Verification items for the finished model (mm, model axes). Face numbers are marked on the shaded views. Give positions to 0.01 mm unless a question says otherwise; leave off trailing zeros. Order: outer loops, then holes, each group sorted by start corner. A loop starts at its lowest first (then second) coordinate and runs counter-clockwise, first axis right, second up. Notation, with made-up numbers: (-35, -23.75) -> (21, -23.75) arc R17 cw to (21, 6.25) -> close; hole circle Ø10 at (5, 27). An arc over 180 degrees is marked (long way). Write each question's results on one line, items separated by ' | '. Start each with the question number.
1. Cross-section at A-A, the plane y = 32.5. Enter the section's corners in (x, z) (3 decimals), then the cut area to 3 significant figures.
2. Depth check by flat-ended pin: pin 1 Ø1.5 at (y, z) = (56, -0.5) entering from +X; pin 2 Ø4 at (y, z) = (60, 2.5) entering from -X; pin 3 Ø5.5 at (x, z) = (7, -6) entering from -Y. Enter the tip coordinate at first touch or a pass-through.
3. Cross-section at C-C, the plane z = -5. Enter the section's corners in (x, y).
4. Cross-section at B-B, the plane x = 2. Enter the section's corners in (y, z).
5. Cross-section at D-D, the plane y = 46. Enter the section's corners in (x, z) (3 decimals), then the cut area to 3 significant figures.
6. Material ranges on L1, parallel to Z at x = 2, y = 43; L2, parallel to Z at x = 46.5, y = 44; L3, parallel to X at y = 30, z = 3.5, recorded low to high. Write a range as from..to.
7. Mould release check, pull along X, two halves, no side actions. Record for the marked faces 1 and 2: +X half, -X half, draft (parallel to the pull), parting line (faces both ways), or undercut.
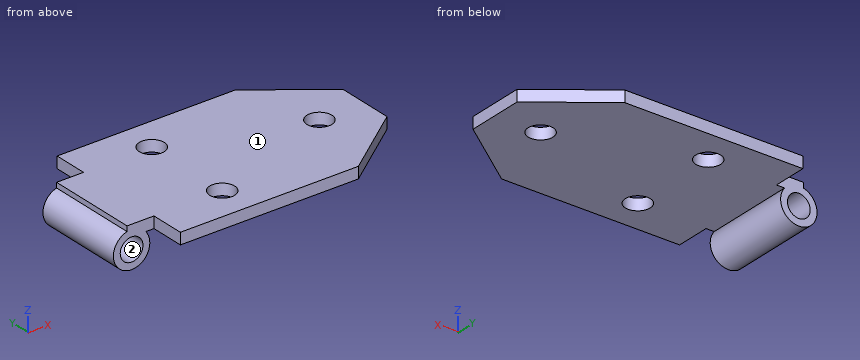
from build123d import *

# Parameters (mm, degrees)
SKETCH1_R               = 5.501178274
BOSS_EXTRUDE1_DEPTH     = 5
SKETCH2_R               = 8
SKETCH2_R_2             = 5
BOSS_EXTRUDE2_DEPTH     = 70
CUT_EXTRUDE2_DEPTH      = 140.531358483
CUT_EXTRUDE2_DEPTH_BACK = 140.531358483
SKETCH4_W               = 17.823798536
SKETCH4_H               = 15


with BuildPart() as part:
    # Sketch1 → Boss-Extrude1 (new body)
    with BuildSketch(Plane.XY):
        Polygon((0, 15), (11.823798536, 15), (11.823798536, 0), (90.043570566, 0), (120, 22.467322075), (120, 47.532677925), (90.043570566, 70), (11.823798536, 70), (11.823798536, 55), (0, 55), align=None)
        with Locations((41.814977969, 55)):
            Circle(SKETCH1_R, mode=Mode.SUBTRACT)
        with Locations((41.814977969, 15)):
            Circle(SKETCH1_R, mode=Mode.SUBTRACT)
        with Locations((100, 35)):
            Circle(SKETCH1_R, mode=Mode.SUBTRACT)
    extrude(amount=BOSS_EXTRUDE1_DEPTH)

    # Sketch2 → Boss-Extrude2 (add)
    with BuildSketch(Plane(origin=(0, 0, 0), x_dir=(1, 0, 0), z_dir=(0, 1, 0))):
        with Locations(Location((2, 5, 0), (0, 0, 270))):
            Circle(SKETCH2_R)
        with Locations(Location((2, 5, 0), (0, 0, 270))):
            Circle(SKETCH2_R_2, mode=Mode.SUBTRACT)
    extrude(amount=BOSS_EXTRUDE2_DEPTH)

    # Sketch4 → Cut-Extrude2 (cut, two sides: drawn at the far end of the back side and taken through both)
    with BuildSketch(Plane.XY.offset(-CUT_EXTRUDE2_DEPTH_BACK)):
        with Locations((2.911899268, 62.5)):
            Rectangle(SKETCH4_W, SKETCH4_H)
        with Locations((2.911899268, 7.5)):
            Rectangle(SKETCH4_W, SKETCH4_H)
    extrude(amount=CUT_EXTRUDE2_DEPTH + CUT_EXTRUDE2_DEPTH_BACK, mode=Mode.SUBTRACT)


solid = part.part
Results below:
1) outline: (0, 2.746) arc R8 ccw (long way) to (8.245, 0) -> (95.1, 0) -> (95.1, 5) -> (0, 5) -> close; (104.9, 0) -> (120, 0) -> (120, 5) -> (104.9, 5) -> close; hole circle Ø10 at (2, -5) | area: 655 mm²
2) pin 1: stops at x = 109.46 | pin 2: stops at x = 11.82 | pin 3: stops at y = 15
3) outline: (-6, 15) -> (-3, 15) -> (-3, 55) -> (-6, 55) -> close; (7, 15) -> (10, 15) -> (10, 55) -> (7, 55) -> close
4) outline: (15, -13) -> (55, -13) -> (55, -10) -> (15, -10) -> close; (15, 0) -> (55, 0) -> (55, 5) -> (15, 5) -> close
5) outline: (0, 2.746) arc R8 ccw (long way) to (8.245, 0) -> (120, 0) -> (120, 5) -> (0, 5) -> close; hole circle Ø10 at (2, -5) | area: 704 mm²
6) L1: z = -13..-10, 0..5 | L2: z = 0..5 | L3: x = 0..97.71, 102.29..120
7) face 1: draft | face 2: undercut
